CAD build for the part. Positions are in the model's coordinates, mm. A direction names the side the tool comes from. Give positions to 0.01 mm unless a question says otherwise; leave off trailing zeros. Write each loop counter-clockwise with the first axis right and the second up, starting at its lowest first coordinate (ties: lowest second). Pieces come first, ordered by that corner, then holes. Notation, with made-up numbers: (13, 21.25) - (37, 21.25) arc R17 ccw to (37, 49.25) - close; hole circle Ø9 at (65.5, 14). An arc over 180 degrees is marked (long way). Answer as a JSON object with one key per item and string values.
from build123d import *

# Parameters (mm, degrees)
F3_DEPTH        = 1.3
F5_START        = -10
F5_DEPTH        = 10
F5_COPIES_COUNT = 6
F6_T4_DEPTH     = 8.638880276
F6_S5_R         = 7.5
F6_T6_DEPTH     = 6
F6_T10_DEPTH    = 8.638880276
F6_S11_R        = 7.5
F6_T12_DEPTH    = 6
F6_T16_DEPTH    = 8.638880276
F6_S17_R        = 7.5
F6_T18_DEPTH    = 6
F6_T22_DEPTH    = 8.638880276
F6_S23_R        = 7.5
F6_T24_DEPTH    = 6
F6_T28_DEPTH    = 8.638880276
F6_S29_R        = 7.5
F6_T30_DEPTH    = 6
F6_T34_DEPTH    = 8.638880276
F6_S35_R        = 7.5
F6_T36_DEPTH    = 6


# Not quite as in the source:
# - a fillet or chamfer that OpenCascade refuses, or shapes differently, is made with other operations: its cross-section is extruded or revolved along the edge and cut away or added
# - a pattern or mirror of a feature is missing from the dataset's text; its kind, count and spacing are read off the source's solid
# - a feature names something its author has since deleted; it is built from what else it names


with BuildPart() as f1:
    # F0 (on Front) → F1 (revolve)
    with BuildSketch(Plane.XZ):
        Polygon((70, 5), (66, 5), (66, 6), (57.5, 6), (57.5, 6.5), (50, 6.5), (50, 7.5), (0, 7.5), (0, 0), (70, 0), align=None)
    revolve(axis=Axis((22.5240401924, 0, 0), (1, 0, 0)))

    # F2 (on face) → F3 (cut)
    with BuildSketch(Plane.YZ.offset(70)):
        with BuildLine():
            ThreePointArc((0.75, 4.9434299833), (0, 5), (-0.75, 4.9434299833))
            Line((-0.75, 4.9434299833), (-0.75, -4.9434299833))
            ThreePointArc((-0.75, -4.9434299833), (0, -5), (0.75, -4.9434299833))
            Line((0.75, -4.9434299833), (0.75, 4.9434299833))
        make_face()
    extrude(amount=-F3_DEPTH, mode=Mode.SUBTRACT)

    # F4 (on face) → F5 (join)
    with BuildSketch(Plane.YZ.offset(50).offset(F5_START)):
        with BuildLine():
            ThreePointArc((-1, 7.4330343737), (0, 7.5), (1, 7.4330343737))
            Line((1, 7.4330343737), (1, 8.3))
            Line((1, 8.3), (-1, 8.3))
            Line((-1, 8.3), (-1, 7.4330343737))
        make_face()
    f5 = extrude(amount=-F5_DEPTH)

    # F5_copies: F5 ×6 about axis
    f5_copies_axis = Axis((0, 0, 0), (1, 0, 0))
    for i in range(1, F5_COPIES_COUNT):
        add(f5.rotate(f5_copies_axis, i * 360 / F5_COPIES_COUNT))

    # F6: chamfer of 0.9 x 1.2853332061 on 6 edges, made by hand


with BuildPart() as f6_tool2:
    # F6_s3 → F6_t4 (new body)
    with BuildSketch(Plane.XZ.offset(-4.319440138)):
        with BuildLine():
            Line((29.9578846671, 7.3705105264), (31.327448539, 8.3294894736))
            Line((31.327448539, 8.3294894736), (31.327448539, 8.3551961377))
            ThreePointArc((31.327448539, 8.3551961377), (30.6637242695, 8.3257066641), (30, 8.3257066641))
            Line((30, 8.3257066641), (29.9742933359, 8.3))
            ThreePointArc((29.9742933359, 8.3), (29.9742933359, 7.8352552632), (29.9321780029, 7.3705105264))
            Line((29.9321780029, 7.3705105264), (29.9578846671, 7.3705105264))
        make_face()
    extrude(amount=F6_T4_DEPTH)

    # F6_s5 → F6_t6 (cut, symmetric)
    with BuildSketch(Plane.YZ.offset(30.6)):
        Circle(F6_S5_R)
    extrude(amount=F6_T6_DEPTH, both=True, mode=Mode.SUBTRACT)


with BuildPart() as f1_1:
    add(f1.part)

    # F6_t1: cut F6_tool2
    add(f6_tool2.part, mode=Mode.SUBTRACT)


with BuildPart() as f6_tool8:
    # F6_s9 → F6_t10 (new body)
    with BuildSketch(Plane.XZ.offset(4.319440138)):
        with BuildLine():
            Line((31.327448539, -8.3294894736), (29.9578846671, -7.3705105264))
            Line((29.9578846671, -7.3705105264), (29.9321780029, -7.3705105264))
            ThreePointArc((29.9321780029, -7.3705105264), (29.9742933359, -7.8352552632), (29.9742933359, -8.3))
            Line((29.9742933359, -8.3), (30, -8.3257066641))
            ThreePointArc((30, -8.3257066641), (30.6637242695, -8.3257066641), (31.327448539, -8.3551961377))
            Line((31.327448539, -8.3551961377), (31.327448539, -8.3294894736))
        make_face()
    extrude(amount=-F6_T10_DEPTH)

    # F6_s11 → F6_t12 (cut, symmetric)
    with BuildSketch(Plane.YZ.offset(30.6)):
        Circle(F6_S11_R)
    extrude(amount=F6_T12_DEPTH, both=True, mode=Mode.SUBTRACT)


with BuildPart() as f1_2:
    add(f1_1.part)

    # F6_t7: cut F6_tool8
    add(f6_tool8.part, mode=Mode.SUBTRACT)


with BuildPart() as f6_tool14:
    # F6_s15 → F6_t16 (new body)
    with BuildSketch(Plane(origin=(0, -2.159720069, 3.7407448896), x_dir=(1, 0, 0), z_dir=(0, 0.5, -0.8660254038))):
        with BuildLine():
            Line((29.9578846671, 7.3705105264), (31.327448539, 8.3294894736))
            Line((31.327448539, 8.3294894736), (31.327448539, 8.3551961377))
            ThreePointArc((31.327448539, 8.3551961377), (30.6637242695, 8.3257066641), (30, 8.3257066641))
            Line((30, 8.3257066641), (29.9742933359, 8.3))
            ThreePointArc((29.9742933359, 8.3), (29.9742933359, 7.8352552632), (29.9321780029, 7.3705105264))
            Line((29.9321780029, 7.3705105264), (29.9578846671, 7.3705105264))
        make_face()
    extrude(amount=F6_T16_DEPTH)

    # F6_s17 → F6_t18 (cut, symmetric)
    with BuildSketch(Plane.YZ.offset(30.6)):
        Circle(F6_S17_R)
    extrude(amount=F6_T18_DEPTH, both=True, mode=Mode.SUBTRACT)


with BuildPart() as f1_3:
    add(f1_2.part)

    # F6_t13: cut F6_tool14
    add(f6_tool14.part, mode=Mode.SUBTRACT)


with BuildPart() as f6_tool20:
    # F6_s21 → F6_t22 (new body)
    with BuildSketch(Plane(origin=(0, 2.159720069, 3.7407448896), x_dir=(1, 0, 0), z_dir=(0, -0.5, -0.8660254038))):
        with BuildLine():
            Line((29.9578846671, 7.3705105264), (31.327448539, 8.3294894736))
            Line((31.327448539, 8.3294894736), (31.327448539, 8.3551961377))
            ThreePointArc((31.327448539, 8.3551961377), (30.6637242695, 8.3257066641), (30, 8.3257066641))
            Line((30, 8.3257066641), (29.9742933359, 8.3))
            ThreePointArc((29.9742933359, 8.3), (29.9742933359, 7.8352552632), (29.9321780029, 7.3705105264))
            Line((29.9321780029, 7.3705105264), (29.9578846671, 7.3705105264))
        make_face()
    extrude(amount=F6_T22_DEPTH)

    # F6_s23 → F6_t24 (cut, symmetric)
    with BuildSketch(Plane.YZ.offset(30.6)):
        Circle(F6_S23_R)
    extrude(amount=F6_T24_DEPTH, both=True, mode=Mode.SUBTRACT)


with BuildPart() as f1_4:
    add(f1_3.part)

    # F6_t19: cut F6_tool20
    add(f6_tool20.part, mode=Mode.SUBTRACT)


with BuildPart() as f6_tool26:
    # F6_s27 → F6_t28 (new body)
    with BuildSketch(Plane(origin=(0, -2.159720069, -3.7407448896), x_dir=(1, 0, 0), z_dir=(0, 0.5, 0.8660254038))):
        with BuildLine():
            Line((29.9578846671, 7.3705105264), (31.327448539, 8.3294894736))
            Line((31.327448539, 8.3294894736), (31.327448539, 8.3551961377))
            ThreePointArc((31.327448539, 8.3551961377), (30.6637242695, 8.3257066641), (30, 8.3257066641))
            Line((30, 8.3257066641), (29.9742933359, 8.3))
            ThreePointArc((29.9742933359, 8.3), (29.9742933359, 7.8352552632), (29.9321780029, 7.3705105264))
            Line((29.9321780029, 7.3705105264), (29.9578846671, 7.3705105264))
        make_face()
    extrude(amount=F6_T28_DEPTH)

    # F6_s29 → F6_t30 (cut, symmetric)
    with BuildSketch(Plane.YZ.offset(30.6)):
        Circle(F6_S29_R)
    extrude(amount=F6_T30_DEPTH, both=True, mode=Mode.SUBTRACT)


with BuildPart() as f1_5:
    add(f1_4.part)

    # F6_t25: cut F6_tool26
    add(f6_tool26.part, mode=Mode.SUBTRACT)


with BuildPart() as f6_tool32:
    # F6_s33 → F6_t34 (new body)
    with BuildSketch(Plane(origin=(0, 2.159720069, -3.7407448896), x_dir=(1, 0, 0), z_dir=(0, -0.5, 0.8660254038))):
        with BuildLine():
            Line((29.9578846671, 7.3705105264), (31.327448539, 8.3294894736))
            Line((31.327448539, 8.3294894736), (31.327448539, 8.3551961377))
            ThreePointArc((31.327448539, 8.3551961377), (30.6637242695, 8.3257066641), (30, 8.3257066641))
            Line((30, 8.3257066641), (29.9742933359, 8.3))
            ThreePointArc((29.9742933359, 8.3), (29.9742933359, 7.8352552632), (29.9321780029, 7.3705105264))
            Line((29.9321780029, 7.3705105264), (29.9578846671, 7.3705105264))
        make_face()
    extrude(amount=F6_T34_DEPTH)

    # F6_s35 → F6_t36 (cut, symmetric)
    with BuildSketch(Plane.YZ.offset(30.6)):
        Circle(F6_S35_R)
    extrude(amount=F6_T36_DEPTH, both=True, mode=Mode.SUBTRACT)


with BuildPart() as f1_6:
    add(f1_5.part)

    # F6_t31: cut F6_tool32
    add(f6_tool32.part, mode=Mode.SUBTRACT)


solid = f1_6.part
Item 1: Probe line 1 (Y direction, x = 5, z = -0.25); line 2 (Y direction, x = 9, z = -1); line 3 (Z direction, x = 33, y = -2.5). List the from-to ranges inside material, lowest first. Write a range as from..to.
Entries:
{"line 1": "-7.5..7.5", "line 2": "-7.43..7.43", "line 3": "-7.07..7.07"}
Item 2: Which spindle directions (+Z, -Z, +X, -X, +Y, -Y) get a long thin tool onto all of the face, cutting with end or side? Do faces 1 (the flat face through (69, -0.75, 0)), 2 (the flat face through (40, -7, -4)), 3 (the flat face through (57.5, 6, -2)), 4 (the flat face through (40, 7, -4)). Say none if no direction does.
Entries:
{"face 1": "+Z, -Z, +X", "face 2": "-Z, +X, -Y", "face 3": "+X", "face 4": "-Z, +X, +Y"}
Item 3: Cut at D-D (y = 4). Give the cut face in (x, z), and give its area (3 significant figures).
Entries:
{"outline": "(0, -6.34) - (50, -6.34) - (50, -5.12) - (57.5, -5.12) - (57.5, -4.47) - (66, -4.47) - (66, -3) - (70, -3) - (70, 3) - (66, 3) - (66, 4.47) - (57.5, 4.47) - (57.5, 5.12) - (50, 5.12) - (50, 6.34) - (0, 6.34) - close", "area": "811 mm2"}
Item 4: Flat gauge pins, fed straight in: P1, Ø0.5, axis at y = -6.5, z = 4.5, coming from the +X side; P2, Ø2, axis at x = 44.5, y = -3.5, coming from the -Z side; P3, Ø5, axis at x = 45, y = -6, coming from the -Z side. Where does each tip first touch, or does it go through?
Entries:
{"P1": "x = 40", "P2": "z = -7.07", "P3": "z = -6.63"}
Item 5: Cut at C-C (y = -3.25). Give the cut face in (x, z), and give its area (4 significant figures).
Entries:
{"outline": "(0, -6.76) - (50, -6.76) - (50, -5.63) - (57.5, -5.63) - (57.5, -5.04) - (66, -5.04) - (66, -3.8) - (70, -3.8) - (70, 3.8) - (66, 3.8) - (66, 5.04) - (57.5, 5.04) - (57.5, 5.63) - (50, 5.63) - (50, 6.76) - (0, 6.76) - close", "area": "876.5 mm2"}
Item 6: Cut at B-B (x = 54.5). Give the cut face in (y, z), and give its area (3 significant figures).
Entries:
{"outline": "circle Ø13 at (0, 0)", "area": "133 mm2"}
Item 7: Cut at A-A (z = 0). Give the cut face in (x, y).
Entries:
{"outline": "(0, -7.5) - (50, -7.5) - (50, -6.5) - (57.5, -6.5) - (57.5, -6) - (66, -6) - (66, -5) - (70, -5) - (70, -0.75) - (68.7, -0.75) - (68.7, 0.75) - (70, 0.75) - (70, 5) - (66, 5) - (66, 6) - (57.5, 6) - (57.5, 6.5) - (50, 6.5) - (50, 7.5) - (0, 7.5) - close"}
